from build123d import *

# Parameters (mm, degrees)
SKETCH1_W           = 49
SKETCH1_H           = 45
BOSS_EXTRUDE1_DEPTH = 15
SKETCH2_W           = 49
SKETCH2_H           = 3
BOSS_EXTRUDE2_DEPTH = 43
BOSS_EXTRUDE3_DEPTH = 3
BOSS_EXTRUDE4_DEPTH = 3


with BuildPart() as part:
    # Sketch1 → Boss-Extrude1 (new body)
    with BuildSketch(Plane.XY):
        with Locations((-2.402173913, 0.366847826)):
            Rectangle(SKETCH1_W, SKETCH1_H)
    extrude(amount=BOSS_EXTRUDE1_DEPTH)

    # Sketch2 → Boss-Extrude2 (add)
    with BuildSketch(Plane.XY.offset(15)):
        with Locations((-2.402173913, -20.633152174)):
            Rectangle(SKETCH2_W, SKETCH2_H)
    extrude(amount=BOSS_EXTRUDE2_DEPTH)

    # Sketch4 → Boss-Extrude3 (add)
    with BuildSketch(Plane.ZY.offset(26.902173913)):
        Polygon((15, -19.133152174), (15, 10.866847826), (50, -19.133152174), align=None)
    extrude(amount=-BOSS_EXTRUDE3_DEPTH)

    # Sketch5 → Boss-Extrude4 (add)
    with BuildSketch(Plane(origin=(22.097826087, 0, 0), x_dir=(0, 0, -1), z_dir=(1, 0, 0))):
        Polygon((-15, -19.133152174), (-15, 10.866847826), (-50, -19.133152174), align=None)
    extrude(amount=-BOSS_EXTRUDE4_DEPTH)


solid = part.part
CAD build for the part. Positions are in the model's coordinates, mm. A direction names the side the tool comes from. Give positions to 0.01 mm unless a question says otherwise; leave off trailing zeros. Loops run counter-clockwise (first coordinate to the right, second up) from the corner with the lowest first, then second, coordinate; pieces in that order, holes last. Notation, with made-up numbers: M 55,-37 L 70,-37 A12 cw 70,-27 Z; hole C 49.25,47 d6. An arc over 180 degrees is marked long. Answer in a Markdown table with one row per item. Add a question column.
Item 1: Mould opens along X. For faces 1 (the face through (-25.423, -3.923, 32.255)), 2 (the face through (19.098, -11, 25)), 3 (the face through (22.098, -4, 17)) say: +X half, -X half, draft (parallel to the pull), parting line (faces both ways), or undercut.
Item 2: Band-saw the part on D-D on z = 51. Give the cut face in (x, y), then the cut area to 3 significant figures.
Item 3: Band-saw the part on C-C on x = 4. Give the cut face in (y, z), then the cut area to 3 significant figures.
Item 4: Probe probe 1 along X at (y, z) = (2, 18.5); probe 2 along Z at (x, y) = (12, 12); probe 3 along Y at (x, z) = (-0.5, 34). List the from-to ranges inside material, lowest first.
Item 5: Drop flat-ended pins along their axis: P1, Ø21, axis at x = 0, y = -5.5, coming from the +Z side; P2, Ø9, axis at y = 3, z = 35, coming from the -X side; P3, Ø1, axis at x = -13, z = 42.5, coming from the +Y side. Give the stop position or say it passes through.
Item 6: Band-saw the part on B-B on z = 25. Give the cut face in (x, y).
Item 7: Tool access for faces 4 (the face through (20.619, -3.923, 32.255)), 5 (the face through (-3, -19.133, 36)): list every direction of +Z, -Z, +X, -X, +Y, -Y with a clear straight run to the whole face (end or side of a thin tool).
Item 8: Band-saw the part on A-A on y = -13.5. Give the cut face in (x, z).
Reply:
| question | item | result |
|---|---|---|
| 1 | face 1 | draft |
| 1 | face 2 | undercut |
| 1 | face 3 | +X half |
| 2 | outline | M -26.9,-22.13 L 22.1,-22.13 L 22.1,-19.13 L -26.9,-19.13 Z |
| 2 | area | 147 mm^2 |
| 3 | outline | M -22.13,0 L 22.87,0 L 22.87,15 L -19.13,15 L -19.13,58 L -22.13,58 Z |
| 3 | area | 804 mm^2 |
| 4 | probe 1 | x = -26.9 to -23.9, 19.1 to 22.1 |
| 4 | probe 2 | z = 0 to 15 |
| 4 | probe 3 | y = -22.13 to -19.13 |
| 5 | P1 | stops at z = 15 |
| 5 | P2 | passes through |
| 5 | P3 | stops at y = -19.13 |
| 6 | outline | M -26.9,-22.13 L 22.1,-22.13 L 22.1,2.3 L 19.1,2.3 L 19.1,-19.13 L -23.9,-19.13 L -23.9,2.3 L -26.9,2.3 Z |
| 7 | face 4 | +Z, +X, -X, +Y |
| 7 | face 5 | +Z, +Y |
| 8 | outline | M -26.9,0 L 22.1,0 L 22.1,43.43 L 19.1,43.43 L 19.1,15 L -23.9,15 L -23.9,43.43 L -26.9,43.43 Z |
